The listing builds one solid part. Answer for the finished solid, in the listing's coordinates (mm). A direction names the side the tool comes from. Give positions to 0.01 mm unless a question says otherwise; leave off trailing zeros. Write each loop counter-clockwise with the first axis right and the second up, starting at its lowest first coordinate (ties: lowest second). Pieces come first, ordered by that corner, then holes. Notation, with made-up numbers: (-9.5, -11) - (-0.5, -11) arc R12 ccw to (-0.5, 3) - close; hole circle Ø5 at (-25.5, -3). An arc over 180 degrees is marked (long way). One line per item, written item: value. Start each with the question number.
from build123d import *

# Parameters (mm, degrees)
F1_DEPTH = 1
F2_W     = 26.5
F2_H     = 19
F3_DEPTH = 1
F4_W     = 10.3
F4_H     = 1.5
F5_DEPTH = 2.5
F6_R     = 0.375
F7_DEPTH = 6


with BuildPart() as f1:
    # F0 (on Front) → F1 (new body)
    with BuildSketch(Plane.XZ):
        with BuildLine():
            ThreePointArc((13.75, 11.75), (13.164214, 13.164214), (11.75, 13.75))
            Line((11.75, 13.75), (-11.75, 13.75))
            ThreePointArc((-11.75, 13.75), (-13.164214, 13.164214), (-13.75, 11.75))
            Line((-13.75, 11.75), (-13.75, -11.75))
            ThreePointArc((-13.75, -11.75), (-13.164214, -13.164214), (-11.75, -13.75))
            Line((-11.75, -13.75), (11.75, -13.75))
            ThreePointArc((11.75, -13.75), (13.164214, -13.164214), (13.75, -11.75))
            Line((13.75, -11.75), (13.75, 11.75))
        make_face()
        with BuildLine():
            Line((-11.35, -10.5), (-8.35, -10.5))
            ThreePointArc((-8.35, -10.5), (-7.642893, -10.792893), (-7.35, -11.5))
            Line((-7.35, -11.5), (-7.35, -12))
            ThreePointArc((-7.35, -12), (-7.642893, -12.707107), (-8.35, -13))
            Line((-8.35, -13), (-11.35, -13))
            ThreePointArc((-11.35, -13), (-12.057107, -12.707107), (-12.35, -12))
            Line((-12.35, -12), (-12.35, -11.5))
            ThreePointArc((-12.35, -11.5), (-12.057107, -10.792893), (-11.35, -10.5))
        make_face(mode=Mode.SUBTRACT)
        with BuildLine():
            Line((7.35, -12), (7.35, -11.5))
            ThreePointArc((7.35, -11.5), (7.642893, -10.792893), (8.35, -10.5))
            Line((8.35, -10.5), (11.35, -10.5))
            ThreePointArc((11.35, -10.5), (12.057107, -10.792893), (12.35, -11.5))
            Line((12.35, -11.5), (12.35, -12))
            ThreePointArc((12.35, -12), (12.057107, -12.707107), (11.35, -13))
            Line((11.35, -13), (8.35, -13))
            ThreePointArc((8.35, -13), (7.642893, -12.707107), (7.35, -12))
        make_face(mode=Mode.SUBTRACT)
        with BuildLine():
            Line((-7.35, 12), (-7.35, 11.5))
            ThreePointArc((-7.35, 11.5), (-7.642893, 10.792893), (-8.35, 10.5))
            Line((-8.35, 10.5), (-11.35, 10.5))
            ThreePointArc((-11.35, 10.5), (-12.057107, 10.792893), (-12.35, 11.5))
            Line((-12.35, 11.5), (-12.35, 12))
            ThreePointArc((-12.35, 12), (-12.057107, 12.707107), (-11.35, 13))
            Line((-11.35, 13), (-8.35, 13))
            ThreePointArc((-8.35, 13), (-7.642893, 12.707107), (-7.35, 12))
        make_face(mode=Mode.SUBTRACT)
        with BuildLine():
            Line((11.35, 10.5), (8.35, 10.5))
            ThreePointArc((8.35, 10.5), (7.642893, 10.792893), (7.35, 11.5))
            Line((7.35, 11.5), (7.35, 12))
            ThreePointArc((7.35, 12), (7.642893, 12.707107), (8.35, 13))
            Line((8.35, 13), (11.35, 13))
            ThreePointArc((11.35, 13), (12.057107, 12.707107), (12.35, 12))
            Line((12.35, 12), (12.35, 11.5))
            ThreePointArc((12.35, 11.5), (12.057107, 10.792893), (11.35, 10.5))
        make_face(mode=Mode.SUBTRACT)
    extrude(amount=-F1_DEPTH)

    # F2 (on face) → F3 (join)
    with BuildSketch(Plane.XZ):
        Rectangle(F2_W, F2_H)
    extrude(amount=F3_DEPTH)

    # F4 (on face) → F5 (join)
    with BuildSketch(Plane(origin=(0, 1, 0), x_dir=(-1, 0, 0), z_dir=(0, 1, 0))):
        with Locations((0, 13)):
            Rectangle(F4_W, F4_H)
    extrude(amount=F5_DEPTH)

    # F6 (on face) → F7 (join)
    with BuildSketch(Plane(origin=(0, 3.5, 0), x_dir=(-1, 0, 0), z_dir=(0, 1, 0))):
        with Locations((-1.25, 13)):
            Circle(F6_R)
        with Locations((-3.75, 13)):
            Circle(F6_R)
        with Locations((1.25, 13)):
            Circle(F6_R)
        with Locations((3.75, 13)):
            Circle(F6_R)
    extrude(amount=F7_DEPTH)


solid = f1.part
Item 1: Each of these flat-tipped pins is pushed along its axis until it touches: pin 1 Ø14 at (x, z) = (-4.5, 0.5) entering from +Y; pin 2 Ø0.5 at (x, y) = (2.5, -0.5) entering from -Z; pin 3 Ø0.8 at (x, y) = (-6, -0.5) entering from +Z; pin 4 Ø1.5 at (y, z) = (3, -1) entering from -X. Where does it stop, or does it pass through?
Item 2: Find section C-C on y = 6.5. Determine the outline of the cut face in (x, z) (3 decimals).
Item 3: The mould has two halves that part along Z. Classify faces 1 (the cylindrical face through (-13.18, 0.49, -13.15)), 2 (the flat face through (5.15, 2, 13)), 3 (the flat face through (9.8, 0.5, -10.5)): +Z half, -Z half, draft (parallel to the pull), parting line (faces both ways), or undercut.
Item 4: Find section D-D on y = 0.5. Give the number of separate pieces and of enclosed holes in the cut face, plus the area to 3 significant figures.
Item 5: Find section B-B on z = 0.25. Determine the outline of the cut face in (x, y), plus the area to 3 significant figures.
Item 6: Straight lines are drawn through the part: line 1 along Y through (x, z) = (3.75, -3); line 2 along Z through (x, y) = (3.5, 2); line 3 along Z through (x, y) = (8.5, -0.25). For each, find the intervals that lie inside material, in ascending order.
Item 7: Find section A-A on x = 2. Determine the outline of the cut face in (y, z), plus the area to 4 significant figures.
Item 8: For faces 4 (the cylindrical face through (-7.635, 0.493, 10.801)), 5 (the flat face through (13.25, -0.5, -0.1)), 6 (the flat face through (-13.25, -0.5, -0.1)), determine the directions among +Z, -Z, +X, -X, +Y, -Y from which every point of the face is accessible in a straight line to the end or side of a thin tool.
Values:
1. pin 1: y = 1
1. pin 2: z = -9.5
1. pin 3: z = 9.5
1. pin 4: through
2. outline: circle Ø0.75 at (-3.75, 13); circle Ø0.75 at (-1.25, 13); circle Ø0.75 at (1.25, 13); circle Ø0.75 at (3.75, 13)
3. face 1: -Z half
3. face 2: draft
3. face 3: undercut
4. separate pieces: 1
4. enclosed holes: 4
4. area: 706 mm^2
5. outline: (-13.75, 0) - (-13.25, 0) - (-13.25, -1) - (13.25, -1) - (13.25, 0) - (13.75, 0) - (13.75, 1) - (-13.75, 1) - close
5. area: 54.0 mm^2
6. line 1: -1 to 1
6. line 2: 12.25 to 13.75
6. line 3: -9.5 to 9.5
7. outline: (-1, -9.5) - (0, -9.5) - (0, -13.75) - (1, -13.75) - (1, 12.25) - (3.5, 12.25) - (3.5, 13.75) - (0, 13.75) - (0, 9.5) - (-1, 9.5) - close
7. area: 50.25 mm^2
8. face 4: +Y, -Y
8. face 5: +Z, -Z, +X, -Y
8. face 6: +Z, -Z, -X, -Y
